```python
from build123d import *

# Parameters (mm, degrees)
PAD002_DEPTH            = 13.5
PAD003_DEPTH            = 1
PAD008_DEPTH            = 1
BODY001_PLACEMENT_ANGLE = -90.0000000001
SKETCH_W                = 150
SKETCH_H                = 13.5
SKETCH_R                = 1.6
PAD_DEPTH               = 4
SKETCH001_W             = 16
SKETCH001_H             = 13.5
PAD001_DEPTH            = 15
FILLET_R                = 10.99
POCKET_DEPTH            = 2.5
SKETCH015_R             = 1.6
POCKET001_DEPTH         = 15.001


with BuildPart() as clip_lm6uu:
    # Sketch003 → Pad002 (new body)
    with BuildSketch(Plane.YZ):
        with BuildLine():
            Line((-8, 0), (-8, -8))
            Line((-8, -8), (8, -8))
            Line((8, 0), (8, -8))
            Line((8, 0), (6.1, 0))
            ThreePointArc((-6.1, 0), (0, -6.1), (6.1, 0))
            ThreePointArc((-4.3133513652, 4.3133513652), (-5.6356651483, 2.3343689374), (-6.1, 0))
            Line((-5.6568542495, 5.6568542495), (-4.3133513652, 4.3133513652))
            ThreePointArc((-5.6568542495, 5.6568542495), (-7.3910362601, 3.0614674589), (-8, 0))
        make_face()
    extrude(amount=PAD002_DEPTH)

    # Sketch002 → Pad003 (join)
    with BuildSketch(Plane.YZ):
        with BuildLine():
            ThreePointArc((-4.1012193309, 4.1012193309), (-2.2195639077, -5.3585012886), (5.8, 0))
            Line((5.8, 0), (6.1, 0))
            ThreePointArc((-4.3133513652, 4.3133513652), (-2.3343689374, -5.6356651483), (6.1, 0))
            Line((-4.1012193309, 4.1012193309), (-4.3133513652, 4.3133513652))
        make_face()
    extrude(amount=PAD003_DEPTH)

    # Sketch013 (on Face5 of Pad003) → Pad008 (join)
    with BuildSketch(Plane.YZ.offset(13.5)):
        with BuildLine():
            ThreePointArc((-4.3133513652, 4.3133513652), (-2.3343689374, -5.6356651483), (6.1, 0))
            Line((5.8, 0), (6.1, 0))
            ThreePointArc((-4.1012193309, 4.1012193309), (-2.2195639077, -5.3585012886), (5.8, 0))
            Line((-4.3133513652, 4.3133513652), (-4.1012193309, 4.1012193309))
        make_face()
    extrude(amount=-PAD008_DEPTH)


with BuildPart() as clip_lm6uu_1:
    # Body001 placement: moved
    add(clip_lm6uu.part.moved(Location((-46, 8.5, 23))).rotate(Axis((-46, 8.5, 23), (0, 0, 1)), BODY001_PLACEMENT_ANGLE))


with BuildPart() as clip_lm6uu_mirror:
    # Part__Mirroring: instance of Clip_LM6UU
    add(clip_lm6uu_1.part.mirror(Plane(origin=(0, 0, 0), x_dir=(0, -1, 0), z_dir=(1, 0, 0))))


with BuildPart() as bedclamping_refined:
    # Sketch → Pad (new body)
    with BuildSketch(Plane.XY):
        with Locations((0, 1.75)):
            Rectangle(SKETCH_W, SKETCH_H)
        with Locations((-70, 0)):
            Circle(SKETCH_R, mode=Mode.SUBTRACT)
        with Locations((-22, 0)):
            Circle(SKETCH_R, mode=Mode.SUBTRACT)
        with Locations((22, 0)):
            Circle(SKETCH_R, mode=Mode.SUBTRACT)
        with Locations((70, 0)):
            Circle(SKETCH_R, mode=Mode.SUBTRACT)
    extrude(amount=PAD_DEPTH)

    # Sketch001 → Pad001 (join)
    with BuildSketch(Plane.XY):
        with Locations((-46, 1.75)):
            Rectangle(SKETCH001_W, SKETCH001_H)
        with Locations((46, 1.75)):
            Rectangle(SKETCH001_W, SKETCH001_H)
    extrude(amount=PAD001_DEPTH)

    # Fillet
    fillet_edges = [bedclamping_refined.edges().sort_by_distance(p)[0] for p in [
        (-54, 1.75, 4),
        (-38, 1.75, 4),
        (38, 1.75, 4),
        (54, 1.75, 4),
    ]]
    fillet(fillet_edges, radius=FILLET_R)

    # Sketch014 → Pocket (cut)
    with BuildSketch(Plane.XY):
        Polygon((-12.5, -3.2331615075), (-9.7, -1.6165807537), (-9.7, 1.6165807537), (-12.5, 3.2331615075), (-15.3, 1.6165807537), (-15.3, -1.6165807537), align=None)
        Polygon((12.5, -3.2331615075), (15.3, -1.6165807537), (15.3, 1.6165807537), (12.5, 3.2331615075), (9.7, 1.6165807537), (9.7, -1.6165807537), align=None)
    extrude(amount=POCKET_DEPTH, mode=Mode.SUBTRACT)

    # Sketch015 → Pocket001 (cut, through all)
    with BuildSketch(Plane.XY):
        with Locations((-12.5, 0)):
            Circle(SKETCH015_R)
        with Locations((12.5, 0)):
            Circle(SKETCH015_R)
    extrude(amount=POCKET001_DEPTH, mode=Mode.SUBTRACT)

    # Fusion: union Clip_LM6UU_Mirror, Clip_LM6UU
    add(clip_lm6uu_mirror.part)
    add(clip_lm6uu_1.part)


solid = bedclamping_refined.part
```
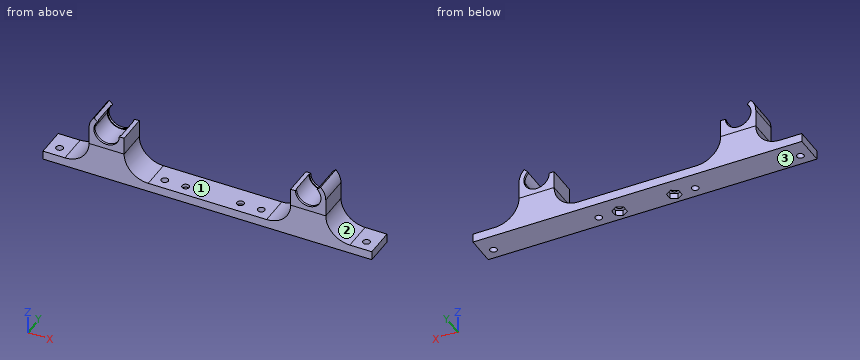
Build history of the part. All positions in model axes, mm. Face numbers are marked on the shaded views. Round coordinates to 2 decimals unless told otherwise and drop trailing zeros. Loops run counter-clockwise (first coordinate to the right, second up) from the corner with the lowest first, then second, coordinate; pieces in that order, holes last.
Item 1: Saw through at A-A (x = -22). List the corners of the cut face in (y, z).
Item 2: Saw through at D-D (x = 46). List the corners of the cut face in (y, z), then the cut area to 3 significant figures.
Item 3: Pin check, flat tips, straight feed: P1, Ø4, axis at y = 1, z = 18, coming from the -X side; P2, Ø1, axis at x = -38.5, y = 1, coming from the +Z side; P3, Ø3, axis at y = -0.5, z = 11, coming from the -X side. Stop position of each tip, or through.
Item 4: Drill centre lines: line 1 along Y through (x, z) = (-70, 1.2); line 2 along Z through (x, y) = (-26.5, 0.75); line 3 along X through (y, z) = (4, 24). Where is each one in solid material? Low to high.
Item 5: Saw through at B-B (y = 6). List the corners of the cut face in (x, z).
Item 6: Two-plate mould, pull along X, no slides. Class the marked faces 1, 2 and 3: released by +X, released by -X, zero draft, split by the parting line, or undercut.
Item 7: Saw through at C-C (z = 7). List the corners of the cut face in (x, y).
Worked answers:
1. outline: (-5, 0) - (-1.6, 0) - (-1.6, 4) - (-5, 4) - close; (1.6, 0) - (8.5, 0) - (8.5, 4) - (1.6, 4) - close
2. outline: (-5, 0) - (8.5, 0) - (8.5, 17.2) - (7.5, 17.2) - (7.5, 16.9) - (-4, 16.9) - (-4, 17.2) - (-5, 17.2) - close
2. area: 229 mm2
3. P1: stops at x = -54
3. P2: stops at z = 23
3. P3: stops at x = -55.47
4. line 1: y = -5 to -1.6, 1.6 to 8.5
4. line 2: z = 0 to 4
4. line 3: x = -53.94 to -52.02, 52.02 to 53.94
5. outline: (-75, 0) - (75, 0) - (75, 4) - (64.99, 4) arc R10.99 cw to (54, 14.99) - (54, 23) arc R8 ccw to (51.66, 28.66) - (50.31, 27.31) arc R6.1 cw (long way) to (39.9, 23) - (38, 23) - (38, 14.99) arc R10.99 cw to (27.01, 4) - (-27.01, 4) arc R10.99 cw to (-38, 14.99) - (-38, 23) - (-39.9, 23) arc R6.1 cw (long way) to (-50.31, 27.31) - (-51.66, 28.66) arc R8 ccw to (-54, 23) - (-54, 14.99) arc R10.99 cw to (-64.99, 4) - (-75, 4) - close
6. face 1: undercut
6. face 2: released by +X
6. face 3: zero draft
7. outline: (-57.44, -5) - (-34.56, -5) - (-34.56, 8.5) - (-57.44, 8.5) - close; (34.56, -5) - (57.44, -5) - (57.44, 8.5) - (34.56, 8.5) - close
